Work out the finished part from the listing and answer in its coordinate system (mm). Coordinates: 2 decimals unless noted, no trailing zeros. Order: outer loops, then holes, each group sorted by start corner. A loop starts at its lowest first (then second) coordinate and runs counter-clockwise, first axis right, second up. Notation, with made-up numbers: M 24,41 L 61,41 A27 cw 61,75 Z; hole C 67.25,67 d10. An arc over 180 degrees is marked long. Use a Markdown table: item, result. Add a question column.
Autodesk Inventor part; units mm, degrees
ref_plane "Work Plane2" through (0, 0, -8101) normal (0, 0, 1) x (1, 0, 0)
ref_plane "Work Plane3" through (2600, 0, 0) normal (1, 0, 0) x (0, 1, 0)
ref_plane "Work Plane4" through (2537.8831, 2179.9067, -2717.5683) normal (-0.6423359, -0.7662012, -0.0184479) x (-0.0374831, 0.0554467, -0.9977578)
sketch "Sketch1" plane through (0, 0, 0) normal (0, 0, 1) x (1, 0, 0)
  arc A0 (4796.3585, -1909.6289) -> (3343.4744, 1121.5056) centre (-3903.1767, -4215.7265) ccw
  line L0 (3236.8192, 1046.7661) -> (3343.5051, 1121.464)
  arc A1 (3228.7635, 1285.3391) -> (1546.1726, 3076.3751) centre (-4110.5601, -3923.7232) ccw
  line L1 (3228.7635, 1285.3391) -> (3122.0787, 1210.6419)
  line L2 (1372.9503, 3176.3452) -> (1308.1705, 3064.1503)
  arc A2 (1372.9503, 3176.3452) -> (93.8576, 4024.2684) centre (-4221.2651, -3873.8147) ccw
  line L3 (1481.3729, 2964.1457) -> (1546.1726, 3076.3751)
  arc A3 (4543.4821, -2147.4888) -> (93.8528, 3844.2289) centre (-4256.4671, -4034.5221) ccw
  line L4 (93.8576, 4024.2684) -> (93.8528, 3844.2289)
  line L5 (1308.1705, 3064.1503) -> (1481.3729, 2964.1457)
  line L6 (3122.0787, 1210.6419) -> (3236.8192, 1046.7661)
  arc A4 (4543.4821, -2147.4888) -> (4796.3585, -1909.6289) centre (4134.8595, -1459.7188) ccw
  point P0 (0, 0)
  dimension "d7" = 800
ref_plane "Work Plane2" through (0, 0, -8101) normal (0, 0, 1) x (1, 0, 0)
ref_plane "Work Plane1" through (0, 0, 0) normal (0, 0, 1) x (1, 0, 0)
sketch "Sketch2" plane through (0, 0, -8101) normal (0, 0, 1) x (1, 0, 0)
  arc A0 (1192.0552, 3508.338) -> (93.8528, 4294.485) centre (-5164.5547, -4211.3454) ccw
  arc A1 (3133.8513, 1483.0798) -> (1365.2603, 3408.338) centre (-5051.6105, -4261.3276) ccw
  arc A2 (4543.6426, -2147.8414) -> (93.8528, 4114.0508) centre (-5207.4444, -4365.1147) ccw
  line L0 (1192.0552, 3508.338) -> (1126.9741, 3395.6142)
  line L1 (1365.2603, 3408.338) -> (1300.1792, 3295.6142)
  line L2 (1126.9741, 3395.6142) -> (1300.1792, 3295.6142)
  line L3 (93.8528, 4294.485) -> (93.8528, 4114.0508)
  line L4 (3027.6129, 1408.6909) -> (3133.8513, 1483.0798)
  line L5 (3142.3282, 1244.8605) -> (3248.5665, 1319.2494)
  line L6 (3027.6129, 1408.6909) -> (3142.3282, 1244.8605)
  arc A3 (4803.6655, -1899.2732) -> (3248.5665, 1319.2494) centre (-4832.968, -4570.4704) ccw
  arc A4 (4543.6426, -2147.8414) -> (4803.6655, -1899.2732) centre (4135.0016, -1460.0824) ccw
  point P0 (0, 0)
loft "Loft1" add profiles "Sketch1", "Sketch2"
ref_plane "Work Plane3" through (2600, 0, 0) normal (1, 0, 0) x (0, 1, 0)
sketch "Sketch3" plane through (2600, 0, 0) normal (1, 0, 0) x (0, 1, 0)
  line L0 (3120.8038, -3828.6818) -> (2179.9067, -2717.5683)
  line L1 (2179.9067, -2717.5683) -> (2281.1646, -4539.693)
  line L2 (2281.1646, -4539.693) -> (3120.8038, -3828.6818)
  line L3 (4534.6211, 332.5956) -> (-2270.5383, 332.5956)
  line L4 (-2270.5383, 332.5956) -> (-2270.5383, -8394.1003)
  line L5 (-2270.5383, -8394.1003) -> (4534.6211, -8394.1003)
  line L6 (4534.6211, -8394.1003) -> (4534.6211, 332.5956)
  point P0 (0, 0)
extrude "Extrusion1" cut sketch "Sketch3" along normal through all both and the other way through all
sketch "Sketch5" plane through (2219.0112, 2281.1646, -4539.693) normal (0, -0.9984595, -0.0554857) x (1, 0, 0)
  line L0 (318.8718, 1824.936) -> (250.4195, 0)
  point P0 (-2219.0112, 4659.2715)
ref_plane "Work Plane4" through (2537.8831, 2179.9067, -2717.5683) normal (-0.6423359, -0.7662012, -0.0184479) x (-0.0374831, 0.0554467, -0.9977578)
sketch "Sketch6" plane through (2537.8831, 2179.9067, -2717.5683) normal (-0.6423359, -0.7662012, -0.0184479) x (-0.0374831, 0.0554467, -0.9977578)
  line L0 (-729.0595, -1938.3665) -> (2085.591, -1938.3665)
  line L1 (2085.591, -1938.3665) -> (2085.591, 179.9667)
  line L2 (2085.591, 179.9667) -> (-729.0595, 179.9667)
  line L3 (-729.0595, 179.9667) -> (-729.0595, -1938.3665)
  point P0 (-2737.216, -722.0143)
extrude "Extrusion2" cut sketch "Sketch6" against normal through all
ref_plane "Work Plane5" through (2537.8831, 2179.9067, -2717.5683) normal (-0.9992973, -0.0020798, 0.0374254) x (-0.0374831, 0.0554467, -0.9977578)
sketch "Sketch7" plane through (2537.8831, 2179.9067, -2717.5683) normal (-0.9992973, -0.0020798, 0.0374254) x (-0.0374831, 0.0554467, -0.9977578)
  line L0 (1826.2193, 0) -> (0, 0)
  line L1 (1201.6643, -877.7967) -> (1826.2193, 0)
  line L2 (0, 0) -> (1201.6643, -877.7967)
  point P0 (-2737.216, 2025.7624)
sketch "Sketch8" plane through (2537.8831, 2179.9067, -2717.5683) normal (-0.6423359, -0.7662012, -0.0184479) x (-0.0374831, 0.0554467, -0.9977578)
  line L0 (1826.2193, 0) -> (0, 0)
  line L1 (1201.6643, -1365.6093) -> (1826.2193, 0)
  line L2 (0, 0) -> (1201.6643, -1365.6093)
  point P0 (-2737.216, -722.0143)
loft "Loft2" add profiles "Sketch7" section 1 edges at (2503.6569, 2230.5357, -3628.6306) (1958.4447, 2700.9842, -4184.1874) (1992.6709, 2650.3553, -3273.125)
sketch "Sketch9" plane through (2537.8831, 2179.9067, -2717.5683) normal (0.9992973, 0.0020798, -0.0374254) x (-0.0374831, 0.0554467, -0.9977578)
  line L0 (1201.6643, 877.7967) -> (0, 0)
  line L1 (1826.2193, 0) -> (0, 0)
  line L2 (1826.2193, 0) -> (1201.6643, 877.7967)
  point P0 (-2737.216, -2025.7624)
ref_plane "Work Plane6" through (2469.4307, 2281.1646, -4539.693) normal (0.9992973, 0.0020798, -0.0374254) x (0.0217303, 0.7814048, 0.623646)
sketch "Sketch10" plane through (2469.4307, 2281.1646, -4539.693) normal (0.9992973, 0.0020798, -0.0374254) x (0.0217303, 0.7814048, 0.623646)
  line L0 (1578.0672, -786.8916) -> (-983.5577, -786.8916)
  line L1 (-983.5577, -786.8916) -> (-983.5577, 1970.9014)
  line L2 (-983.5577, 1970.9014) -> (1578.0672, 1970.9014)
  line L3 (1578.0672, 1970.9014) -> (1578.0672, -786.8916)
  point P0 (994.987, 4892.7146)
extrude "Extrusion3" cut sketch "Sketch10" against normal through all
sketch "Sketch11" plane through (2469.4307, 2281.1646, -4539.693) normal (0.9992973, 0.0020798, -0.0374254) x (0.0217303, 0.7814048, 0.623646)
  line L0 (1027.6784, 44.8475) -> (1011.4833, 1341.5246)
  line L1 (1011.4833, 1341.5246) -> (103.4312, 65.2798)
  line L2 (103.4312, 65.2798) -> (1027.6784, 44.8475)
  line L3 (960.9484, 1557.5799) -> (-216.8429, -97.7765)
  line L4 (960.9484, 1557.5799) -> (1128.2932, 1792.779)
  line L5 (1128.2932, 1585.7882) -> (1128.2932, 1792.779)
  line L6 (-69.5683, -97.7765) -> (-216.8429, -97.7765)
  line L7 (1027.6784, -97.7765) -> (1046.3487, -386.6685)
  line L8 (1182.7704, -360.1846) -> (1182.7704, -431.4012)
  arc A0 (1046.3487, -386.6685) -> (1182.7704, -431.4012) centre (1192.5364, -171.2284) ccw
  line L9 (1394.5704, -97.7765) -> (1471.9375, -97.7765)
  line L10 (1171.1456, 55.0636) -> (1464.8769, 44.8475)
  line L11 (1471.9375, -97.7765) -> (1528.8489, -97.7765)
  arc A1 (1528.8489, -97.7765) -> (1464.8769, 44.8475) centre (1251.9333, -136.3242) ccw
  line L12 (1128.2932, 1585.7882) -> (1171.1456, 55.0636)
  line L13 (1175.4243, -97.7765) -> (1182.7704, -360.1846)
  line L14 (-69.5683, -97.7765) -> (1027.6784, -97.7765)
  line L15 (1175.4243, -97.7765) -> (1394.5704, -97.7765)
  point P0 (994.987, 4892.7146)
  point P1 (1077.3097, 0)
  point P2 (1058.7249, 1488.0116)
  point P3 (0, 0)
extrude "Extrusion4" add sketch "Sketch11" against normal blind 150
properties part number "panel_block_03" material "Wood (Maple)"
(1) A cutting plane is placed at A-A on y = 2783. Write down the section's boundary in (x, z).
(2) Given P1, Ø1, axis at x = 2424.5, y = 2270.5, coming from the -Z side; P2, Ø6, axis at x = 2474.5, y = 2453, coming from the +Z side; P3, Ø8, axis at x = 2461, z = -3991.5, coming from the -Y side, each flat-ended and moving along its own axis, determine where each tip first touches the part or whether it passes through.
(3) The mould has two halves that part along Y. Classify faces 1 (the flat face through (2429.54, 2277.065, -3629.106)), 2 (the cylindrical face through (2406.9, 3409.8, -4171)): pulls with the +Y half, pulls with the -Y half, needs draft (parallel to the pull), parting line crosses it, or undercut.
(4) A cutting plane is placed at B-B on y = 2280.5. Write down the section's boundary in (x, z).
(5) Straight lines are drawn through the part: line 1 (Z direction, x = 2393, y = 2622); line 2 (Z direction, x = 2416, y = 2577.5); line 3 (Y direction, x = 2368, z = -3768.5). For each, find the intervals that lie inside material, in ascending order.
(6) A cutting plane is placed at C-C on z = -2646. Write down the section's boundary in (x, y), plus the area to 3 significant figures.
From the geometry:
| question | item | result |
|---|---|---|
| 1 | outline | M 2328.82,-4258.35 L 2478.7,-4264.21 L 2485.9,-4072.11 L 2336.01,-4066.26 Z; M 2356.27,-3525.3 L 2506.18,-3530.53 L 2514.12,-3318.47 L 2364.21,-3313.22 Z |
| 2 | P1 | stops at z = -4672.08 |
| 2 | P2 | stops at z = -2922.98 |
| 2 | P3 | stops at y = 2130.29 |
| 3 | face 1 | undercut |
| 3 | face 2 | pulls with the +Y half |
| 4 | outline | M 2314.84,-4659.4 L 2464.73,-4665.26 L 2501.22,-3690.92 L 2351.11,-3690.92 Z; M 2380.27,-2912.4 L 2530.18,-2917.63 L 2537.41,-2724.59 L 2387.5,-2719.34 Z |
| 5 | line 1 | z = -4389.53 to -4191.42, -3329.94 to -3123.69 |
| 5 | line 2 | z = -4426 to -4226.3, -3276.39 to -3071.83 |
| 5 | line 3 | y = 2118.12 to 2284.81, 2981.79 to 3397.85 |
| 6 | outline | M 2390.38,2218.44 L 2390.72,2055.74 L 2540.82,2055.74 L 2540.49,2214.01 Z |
| 6 | area | 24,100 mm2 |
